```python
from build123d import *

# Parameters (mm, degrees)
F2_R            = 5
F3_DEPTH        = 0.5
F3_COPIES_COUNT = 6


# Not quite as in the source:
# - a pattern or mirror of a feature is missing from the dataset's text; its kind, count and spacing are read off the source's solid


with BuildPart() as f1:
    # F0 (on Top) → F1 (revolve)
    with BuildSketch(Plane.XY):
        with BuildLine():
            Line((0, 6), (0, 0))
            Line((0, 0), (51, 0))
            Line((51, 0), (51, 1.3443025184))
            ThreePointArc((51, 1.3443025184), (50.5372887774, 2.6236551731), (49.363256785, 3.3110369967))
            ThreePointArc((49.363256785, 3.3110369967), (34.7430608343, 5.3263557546), (20, 6))
            Line((20, 6), (0, 6))
        make_face()
    revolve(axis=Axis((0, 3, 0), (0, 1, 0)))

    # F2 (on face) → F3 (cut)
    with BuildSketch(Plane.XZ):
        with Locations((39, 0)):
            Circle(F2_R)
    f3 = extrude(amount=-F3_DEPTH, mode=Mode.SUBTRACT)

    # F3_copies: F3 ×6 about axis
    f3_copies_axis = Axis((0, 0, 0), (0, 1, 0))
    for i in range(1, F3_COPIES_COUNT):
        add(f3.rotate(f3_copies_axis, i * 360 / F3_COPIES_COUNT), mode=Mode.SUBTRACT)


solid = f1.part
```
Geometry: final body of the model. Coordinates: model frame, mm. A direction names the side the tool comes from. Coordinates: 2 decimals unless noted, no trailing zeros. Use CSV: the item, a comma, the result in double quotes. Start each with the question number.
1. Reachability of faces 1 (the face through (23.468, 0.246, 36.817)), 2 (the face through (1, 0, -1)) from +Z, -Z, +X, -X, +Y, -Y: full face, straight path, thin tool, end or side. Return the list, or none.
2. Mould query, pull axis X, two halves, no side actions, for faces 3 (the face through (0, 6, 0)), 4 (the face through (-20, 0.5, 34)), 5 (the face through (-11.056, 0.682, 49.787)). Classes: pulls with the +X half, pulls with the -X half, needs draft (parallel to the pull), parting line crosses it, or undercut.
3. Ray query, probe 1 along Z at (x, y) = (-19.5, 0.3) (3 decimals); probe 2 along Y at (x, z) = (-10, -20); probe 3 along X at (y, z) = (2.75, -28). Return the intervals inside material, ascending.
4. First-contact query: P1, Ø5, axis at x = -19.5, z = -32, coming from the -Y side; P2, Ø2, axis at x = -26, y = 1.5, coming from the -Z side; P3, Ø12, axis at x = -13.5, z = -31, coming from the +Y side. Flat tips, straight axial feed; report the tip coordinate or a pass-through.
Entries:
1,face 1,"-Y"
1,face 2,"+Z, -Z, +X, -X, -Y"
2,face 3,"needs draft"
2,face 4,"undercut"
2,face 5,"parting line crosses it"
3,probe 1,"-47.125 to -38.775, -28.775 to 28.775, 38.775 to 47.125"
3,probe 2,"0 to 5.98"
3,probe 3,"-41.93 to 41.93"
4,P1,"y = 0.5"
4,P2,"z = -44.45"
4,P3,"y = 5.81"
